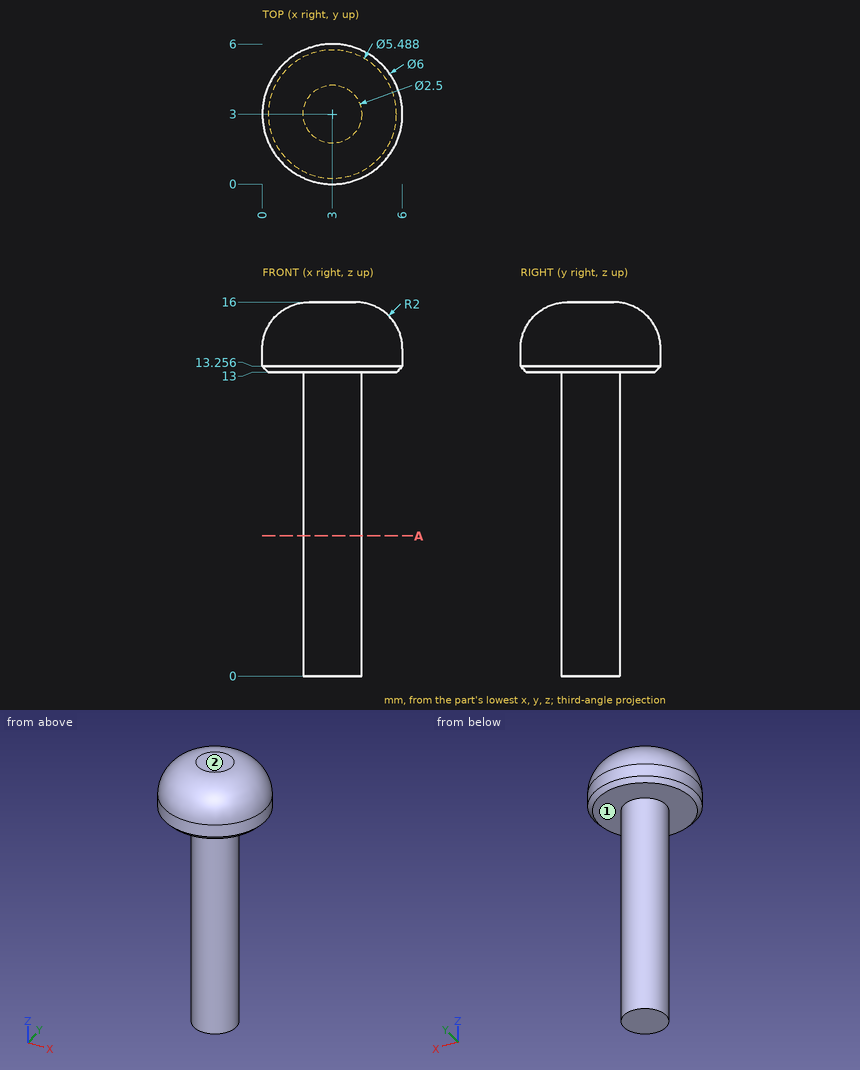
Design review of the part shown in the three views and the two pictorial views. Dimensions are in mm from the part's minimum x, y and z. A direction names the side the tool comes from. Round coordinates to 2 decimals unless told otherwise and drop trailing zeros. Loops run counter-clockwise (first coordinate to the right, second up) from the corner with the lowest first, then second, coordinate; pieces in that order, holes last. Notation, with made-up numbers: (35.5, 59) - (39.5, 59) arc R22 ccw to (39.5, 95) - close; hole circle Ø6 at (18, -21.5). An arc over 180 degrees is marked (long way). One line per item, written item: value. Start each with the question number.
Item 1: Clearance check with flat-ended pins moving along their axes: pin 1 Ø1 at (x, z) = (1, 11.5) entering from +Y; pin 2 Ø2 at (y, z) = (3.5, 11) entering from -X; pin 3 Ø1.5 at (y, z) = (4.5, 9) entering from +X; pin 4 Ø1.5 at (x, z) = (2, 11) entering from -Y. State where each tip first meets the part, or that it passes through.
Item 2: Take a section at A-A (z = 6). Give the boundary of the cut face in (x, y), plus the area to 3 significant figures.
Item 3: For L1, parallel to Y at x = 3, z = 9; L2, parallel to Z at x = 3.25, y = 4.1; L3, parallel to Y at x = 2.25, z = 1, list the stretches that pass through material, from the lowest coordinate up.
Item 4: For the marked faces 1 and 2, list the 3-axis set-ups (+Z, -Z, +X, -X, +Y, -Y) from which the entire face can be reached by the end or side of a thin tool; tool diameter is ignored.
Answer below:
1. pin 1: passes through
1. pin 2: stops at x = 1.75
1. pin 3: stops at x = 4
1. pin 4: stops at y = 1.78
2. outline: circle Ø2.5 at (3, 3)
2. area: 4.91 mm2
3. L1: y = 1.75 to 4.25
3. L2: z = 0 to 16
3. L3: y = 2 to 4
4. face 1: -Z
4. face 2: +Z, +X, -X, +Y, -Y
